The drawing under review shows one solid part. Ordinate dimensions are in mm from its lowest x, y, z. Coordinates: 2 decimals unless noted, no trailing zeros. Loops run counter-clockwise (first coordinate to the right, second up) from the corner with the lowest first, then second, coordinate; pieces in that order, holes last. Notation, with made-up numbers: M -30.5,-33 L 15.5,-33 A23 cw 15.5,2 Z; hole C 77,-38.75 d3. An arc over 180 degrees is marked long. Answer as a JSON object with one key per item and string values. Group by question number.
1. Consider section D-D (y = 35). State the section outline as (x, z) points.
2. To check wall thickness, follow probe 1 along Y at (x, z) = (50, 7); probe 2 along Y at (x, z) = (25, 6); probe 3 along X at (y, z) = (37, 0.75). State the ranges of each line that lie inside material, in increasing order.
3. Consider section C-C (y = 30). State the section outline as (x, z) points, then the cut area to 3 significant figures.
4. Consider section A-A (x = 25). State the section outline as (y, z) points.
5. Draft analysis for pull direction X (two halves, no side actions). For the marked faces 1, 2, 3 and 4, state which applies: +X half, -X half, draft (parallel to the pull), parting line (faces both ways), or undercut.
6. Consider section B-B (z = 6.75). State the section outline as (x, y) points.
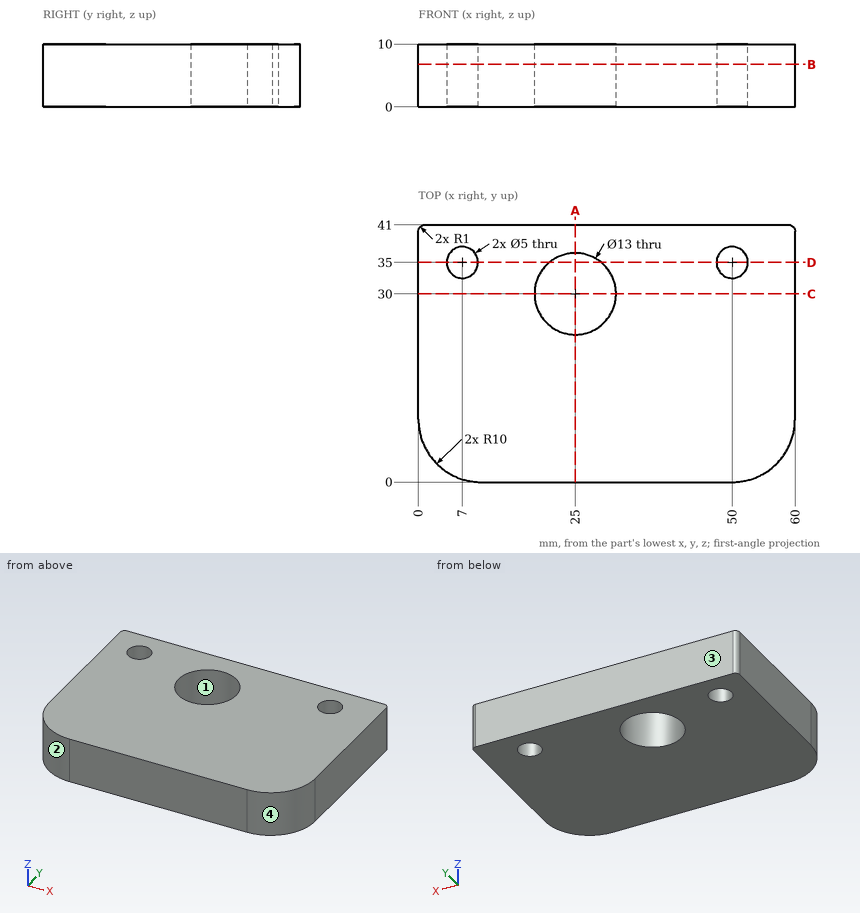
Findings below:
{
 "1": {"outline": "M 0,0 L 4.5,0 L 4.5,10 L 0,10 Z; M 9.5,0 L 20.85,0 L 20.85,10 L 9.5,10 Z; M 29.15,0 L 47.5,0 L 47.5,10 L 29.15,10 Z; M 52.5,0 L 60,0 L 60,10 L 52.5,10 Z"},
 "2": {"probe 1": "y = 0 to 32.5, 37.5 to 41", "probe 2": "y = 0 to 23.5, 36.5 to 41", "probe 3": "x = 0 to 5.5, 8.5 to 48.5, 51.5 to 60"},
 "3": {"outline": "M 0,0 L 18.5,0 L 18.5,10 L 0,10 Z; M 31.5,0 L 60,0 L 60,10 L 31.5,10 Z", "area": "470 mm^2"},
 "4": {"outline": "M 0,0 L 23.5,0 L 23.5,10 L 0,10 Z; M 36.5,0 L 41,0 L 41,10 L 36.5,10 Z"},
 "5": {"face 1": "undercut", "face 2": "-X half", "face 3": "draft", "face 4": "+X half"},
 "6": {"outline": "M 0,10 A10 ccw 10,0 L 50,0 A10 ccw 60,10 L 60,40 A1 ccw 59,41 L 1,41 A1 ccw 0,40 Z; hole C 7,35 d5; hole C 25,30 d13; hole C 50,35 d5"}
}
